Autodesk Inventor part; units mm, degrees
ref_plane "Arbeitsebene2" through (0, 0, 0) normal (0, 0, 1) x (1, 0, 0)
ref_plane "YZ Plane" through (0, 0, 0) normal (1, 0, 0) x (0, 1, 0)
ref_plane "XZ Plane" through (0, 0, 0) normal (0, 1, 0) x (-1, 0, 0)
ref_plane "Arbeitsebene1" through (0, 0, 0) normal (0, 0, 1) x (1, 0, 0)
sketch "Skizze1" plane through (0, 0, 0) normal (0, 0, 1) x (1, 0, 0)
  line L0 (26, 19) -> (14, 19)
  line L1 (14, 19) -> (14, 0)
  line L2 (14, 0) -> (26, 0)
  line L3 (26, 0) -> (26, 19)
  line L4 (0, 0) -> (40, 0)
  line L5 (40, 0) -> (40, 42)
  line L6 (0, 42) -> (40, 42)
  line L7 (0, 0) -> (0, 42)
  line L8 (40, 0) -> (3, 0)
  line L9 (3, 0) -> (3, 27)
  line L10 (3, 27) -> (40, 27)
  line L11 (40, 27) -> (40, 0)
  dimension "d0" = 37
  dimension "d1" = 27
extrude "Extrusion1" add sketch "Skizze1" along normal blind 3 contours L0 L1 L4 L9 L10 L5 L3
sketch "Skizze2" plane through (0, 0, 3) normal (0, 0, 1) x (1, 0, 0)
  line L0 (14, 0) -> (14, 19)
  line L1 (14, 19) -> (26, 19)
  line L2 (26, 19) -> (26, 0)
  line L3 (26, 0) -> (40, 0)
  line L4 (40, 0) -> (40, 27)
  line L5 (40, 27) -> (3, 27)
  line L6 (3, 27) -> (3, 0)
  line L7 (3, 0) -> (14, 0)
  line L8 (9, 29.5) -> (31, 29.5)
  line L9 (31, 29.5) -> (31, -10.5)
  line L10 (31, -10.5) -> (9, -10.5)
  line L11 (9, -10.5) -> (9, 29.5)
  line L12 (9, 29.5) -> (31, -10.5) construction
  line L13 (31, 29.5) -> (9, -10.5) construction
  point P0 (0, 0)
  point P1 (20, 9.5)
  dimension "d4" = 22
  dimension "d5" = 40
extrude "Extrusion2" add sketch "Skizze2" along normal blind 5 contours L7 L11 L5 L9 L3 L2 L1 L0 | L0 L1 L2 L3 L9 L10 L11 L7 | L11 L8 L9 L5
sketch "Skizze3" plane through (0, 0, 8) normal (0, 0, 1) x (1, 0, 0)
  line L0 (14, 0) -> (14, 19)
  line L1 (14, 19) -> (26, 19)
  line L2 (26, 19) -> (26, 0)
  line L3 (14, 0) -> (26, 0)
  circle A0 centre (20, 9.5) radius 9.5
  point P0 (0, 0)
ref_plane "Arbeitsebene2" through (0, 0, 0) normal (0, 0, 1) x (1, 0, 0)
extrude "Extrusion3" cut sketch "Skizze3" against normal up to surface (8 mm away) contours A0 L0 | L0 A0 L2 | L2 A0
properties part number "04_LED_Holder"
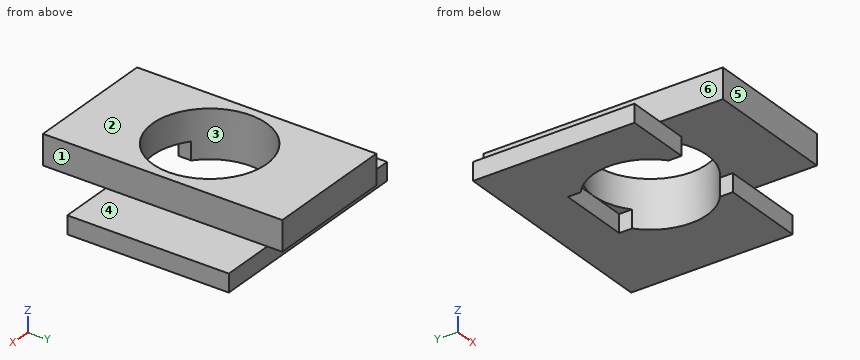
Geometry check sheet. Reference: the model listing, model coordinates, mm. Face numbers are marked on the shaded views. A direction names the side the tool comes from. Give positions to 0.01 mm unless a question says otherwise; leave off trailing zeros. Write each loop counter-clockwise with the first axis right and the second up, starting at its lowest first coordinate (ties: lowest second). Pieces come first, ordered by that corner, then holes. Notation, with made-up numbers: (85.25, 51.25) - (104.25, 51.25) arc R22 ccw to (104.25, 89.25) - close; hole circle Ø3 at (-2.75, -16.5). An arc over 180 degrees is marked (long way). Put each result on its own line as item: value.
1. Draft check along X on the marked faces 1, 2 and 3. Enter one of: +X half, -X half, draft (parallel to the pull), parting line (faces both ways), or undercut.
Ans:
face 1: +X half
face 2: draft
face 3: undercut
2. Set-up check for the marked faces 4, 5 and 6: record each of +Z, -Z, +X, -X, +Y, -Y from which the full face is reachable in a straight line by a thin tool's end or side.
Ans:
face 4: +Z, +X, +Y, -Y
face 5: +Z, -Z, +X, -X, -Y
face 6: +Z, -X, +Y, -Y
3. Sectioned sample at B-B, the plane z = 3.5. Enter the section's corners in (x, y).
Ans:
outline: (9, -10.5) - (31, -10.5) - (31, 29.5) - (9, 29.5) - close; hole circle Ø19 at (20, 9.5)
4. Go/stop test with flat-tipped pins: pin 1 (1 mm diameter, centred on y = 11.5, z = 4, fed in from +X); pin 2 (2 mm diameter, centred on x = 32.5, y = 3, fed in from +Z); pin 3 (0.6 mm diameter, centred on x = 22, y = 18, fed in from -Z); pin 4 (1.7 mm diameter, centred on x = 16.5, y = 18, fed in from -Z). Record where each tip stops, or that it passes through.
Ans:
pin 1: stops at x = 31
pin 2: stops at z = 3
pin 3: passes through
pin 4: stops at z = 3
5. Thickness scan on line 1 (X direction, y = 9.5, z = 5.5); line 2 (X direction, y = 9.5, z = 2.5); line 3 (Z direction, x = 37.5, y = 17.5). Record the ranges inside material, lowest first.
Ans:
line 1: x = 9 to 10.5, 29.5 to 31
line 2: x = 3 to 10.5, 29.5 to 40
line 3: z = 0 to 3
6. Sectioned sample at D-D, the plane y = 25. Enter the section's corners in (x, z), plus the area to 3 significant figures.
Ans:
outline: (3, 0) - (40, 0) - (40, 3) - (31, 3) - (31, 8) - (9, 8) - (9, 3) - (3, 3) - close
area: 221 mm²
7. Sectioned sample at A-A, the plane y = 9.5. Enter the section's corners in (x, z), plus the area to 3 significant figures.
Ans:
outline: (3, 0) - (10.5, 0) - (10.5, 8) - (9, 8) - (9, 3) - (3, 3) - close; (29.5, 0) - (40, 0) - (40, 3) - (31, 3) - (31, 8) - (29.5, 8) - close
area: 69.0 mm²
